from build123d import *

# Parameters (mm, degrees)
SKETCH1_R           = 5.159375
BOSS_EXTRUDE1_DEPTH = 76.2
SKETCH2_R           = 5.582507509
SKETCH2_R_2         = 4.95
CUT_EXTRUDE1_DEPTH  = 12.7
CUT_EXTRUDE2_DEPTH  = 15.24
SKETCH5_R           = 6.855394903
SKETCH5_R_2         = 4.7625
CUT_EXTRUDE3_DEPTH  = 9.525


with BuildPart() as part:
    # Sketch1 → Boss-Extrude1 (new body)
    with BuildSketch(Plane(origin=(0, 0, 0), x_dir=(1, 0, 0), z_dir=(0, 1, 0))):
        with Locations(Location((0, 0, 0), (0, 0, 90))):
            Circle(SKETCH1_R)
    extrude(amount=BOSS_EXTRUDE1_DEPTH)

    # Sketch2 → Cut-Extrude1 (cut)
    with BuildSketch(Plane(origin=(0, 76.2, 0), x_dir=(1, 0, 0), z_dir=(0, 1, 0))):
        Circle(SKETCH2_R)
        with Locations(Location((0, 0, 0), (0, 0, 270))):
            Circle(SKETCH2_R_2, mode=Mode.SUBTRACT)
    extrude(amount=-CUT_EXTRUDE1_DEPTH, mode=Mode.SUBTRACT)

    # Sketch4 → Cut-Extrude2 (cut)
    with BuildSketch(Plane(origin=(4747.84892855, 34.473117596, 51.91521842), x_dir=(-1, 0, 0), z_dir=(0, -1, 0))):
        Polygon((4747.84892855, 56.48021842), (4739.672253117, 56.48021842), (4739.672253117, 59.680433841), (4755.943170737, 59.680433841), (4755.943170737, 56.48021842), align=None)
    extrude(amount=-CUT_EXTRUDE2_DEPTH, mode=Mode.SUBTRACT)

    # Sketch5 → Cut-Extrude3 (cut)
    with BuildSketch(Plane.XZ):
        Circle(SKETCH5_R)
        with Locations(Location((0, 0, 0), (0, 0, 270))):
            Circle(SKETCH5_R_2, mode=Mode.SUBTRACT)
    extrude(amount=-CUT_EXTRUDE3_DEPTH, mode=Mode.SUBTRACT)


solid = part.part
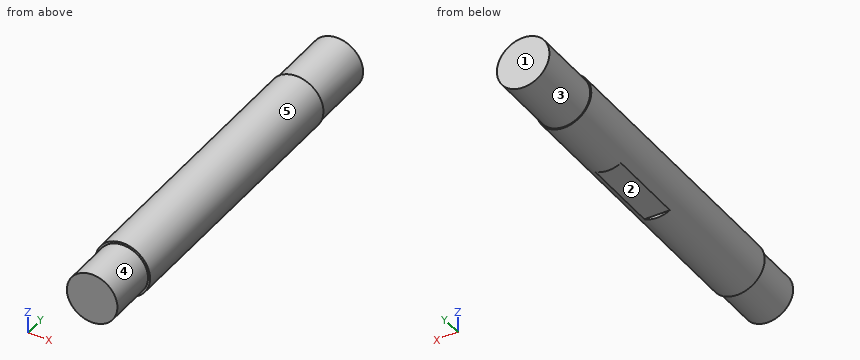
The listing builds one solid part. Answer for the finished solid, in the listing's coordinates (mm). Face numbers are marked on the shaded views. A direction names the side the tool comes from. Give positions to 0.01 mm unless a question says otherwise; leave off trailing zeros. Write each loop counter-clockwise with the first axis right and the second up, starting at its lowest first coordinate (ties: lowest second). Pieces come first, ordered by that corner, then holes.
Item 1: Section C-C, the plane y = 36.5 is taken. Write down the section's boundary in (x, z) (3 decimals).
Item 2: Find the intervals of material crossed by line 1 along Z through (x, y) = (-0.25, 24.5); line 2 along Y through (x, z) = (-3.75, 3) (3 decimals); line 3 along Z through (x, y) = (3, 72), in increasing order.
Item 3: Which of the six approach directions +Z, -Z, +X, -X, +Y, -Y give full straight-line access (tool end or side, diameter ignored) to the marked faces 4 and 5?
Item 4: Section D-D, the plane x = -3.75 is taken. Write down the section's boundary in (y, z) (3 decimals), plus the area to 3 significant figures.
Item 5: Determine the mould class of the marked faces 1, 2 and 3 for opening direction Y: released by +Y, released by -Y, zero draft, split by the parting line, or undercut.
Item 6: Flat-ended cylindrical pins translate along their axes: P1, Ø1.5, axis at y = 32, z = -1, coming from the -X side; P2, Ø5.5, axis at x = -0.5, y = 40, coming from the -Z side (3 decimals). Find the tip coordinate at first contact, or state that the pin passes through.
Completed:
1. outline: (-2.404, -4.565) - (2.404, -4.565) arc R5.159 ccw (long way) to start
2. line 1: z = -5.15 to 5.15
2. line 2: y = 9.525 to 76.2
2. line 3: z = -3.94 to 3.94
3. face 4: -Y
3. face 5: +Y, -Y
4. outline: (0, -2.936) - (9.525, -2.936) - (9.525, -3.544) - (63.5, -3.544) - (63.5, -3.231) - (76.2, -3.231) - (76.2, 3.231) - (63.5, 3.231) - (63.5, 3.544) - (9.525, 3.544) - (9.525, 2.936) - (0, 2.936) - close
4. area: 521 mm2
5. face 1: released by +Y
5. face 2: undercut
5. face 3: zero draft
6. P1: stops at x = -5.15
6. P2: stops at z = -4.565
